Model file for the job. Use its own axes, mm. A direction names the side the tool comes from. Give positions to 0.01 mm unless a question says otherwise; leave off trailing zeros. Loops run counter-clockwise (first coordinate to the right, second up) from the corner with the lowest first, then second, coordinate; pieces in that order, holes last. Notation, with made-up numbers: M -20,-24.5 L 33,-24.5 A16 ccw 33,-8.5 Z; hole C -10,65 d8. An arc over 180 degrees is marked long. Use CSV: the item, a comma, the result in double quotes. Start each with the question number.
(1) Flat gauge pins, fed straight in: P1, Ø20, axis at y = 54, z = 58.5, coming from the -X side; P2, Ø5, axis at y = 65, z = 67, coming from the +X side; P3, Ø6, axis at x = 40.5, y = 64.5, coming from the +Z side. Where does each tip first touch, or does it go through?
(2) Two-plate mould, pull along Y, no slides. Class faces 6 (the face through (50, 0, 50)), 7 (the face through (50, 40, 57)), 8 (the face through (88, 32, 49)), 9 (the face through (80, 5, 50)): pulls with the +Y half, pulls with the -Y half, needs draft (parallel to the pull), parting line crosses it, or undercut.
(3) Slice it at D-D on z = 17.5. List the corners of the cut face in (x, y), and give its area (3 significant figures).
(4) Slice it at B-B on y = 43.5. List the corners of the cut face in (x, z), and give its area (3 significant figures).
(5) Tool access for faces 1 (the face through (50, 60, 57)), 2 (the face through (20, 65, 41)), 3 (the face through (83, 10, 51)), 4 (the face through (80, 64, 41)), 5 (the face through (20, 5, 50)): list every direction of +Z, -Z, +X, -X, +Y, -Y with a clear straight run to the whole face (end or side of a thin tool).
(6) Wall check: line 1 along Y through (x, z) = (34.5, 39); line 2 along X through (y, z) = (60.5, 67.5); line 3 along Z through (x, y) = (50.5, 43.5). Give the ranges that are in metal, low to high. Write a range as from..to.
(7) Slice it at C-C on x = 41. List the corners of the cut face in (y, z).
(8) Slice it at A-A on z = 94. List the corners of the cut face in (x, y), and give its area (3 significant figures).
```python
from build123d import *

# Parameters (mm, degrees)
SKETCH1_W           = 100
SKETCH1_H           = 80
BOSS_EXTRUDE2_DEPTH = 100
SKETCH2_W           = 20
SKETCH2_H           = 10
CUT_EXTRUDE1_DEPTH  = 100
CUT_EXTRUDE2_DEPTH  = 100
SKETCH4_W           = 15
SKETCH4_H           = 10
CUT_EXTRUDE5_DEPTH  = 100
SKETCH7_R           = 35
CUT_EXTRUDE16_DEPTH = 20
BOSS_EXTRUDE3_DEPTH = 40
CUT_EXTRUDE17_DEPTH = 10
SKETCH18_W          = 60
SKETCH18_H          = 20
CUT_EXTRUDE22_DEPTH = 75


with BuildPart() as part:
    # Sketch1 → Boss-Extrude2 (new body)
    with BuildSketch(Plane.XY):
        with Locations((50, 40)):
            Rectangle(SKETCH1_W, SKETCH1_H)
    extrude(amount=BOSS_EXTRUDE2_DEPTH)

    # Sketch2 → Cut-Extrude1 (cut)
    with BuildSketch(Plane.XY):
        Polygon((0, 80), (20, 80), (20, 40), (0, 20), align=None)
        with Locations((10, 5)):
            Rectangle(SKETCH2_W, SKETCH2_H)
        with Locations((90, 5)):
            Rectangle(SKETCH2_W, SKETCH2_H)
        Polygon((80, 80), (100, 80), (100, 20), (80, 40), align=None)
    extrude(amount=CUT_EXTRUDE1_DEPTH, mode=Mode.SUBTRACT)

    # Sketch3 → Cut-Extrude2 (cut)
    with BuildSketch(Plane(origin=(0, 80, 0), x_dir=(1, 0, 0), z_dir=(0, 1, 0))):
        with BuildLine():
            Line((0, 0), (0, -50))
            ThreePointArc((0, -50), (14.644660941, -14.644660941), (50, 0))
            Line((50, 0), (0, 0))
        make_face()
        with BuildLine():
            Line((100, 0), (50, 0))
            ThreePointArc((50, 0), (85.355339059, -14.644660941), (100, -50))
            Line((100, -50), (100, 0))
        make_face()
        with BuildLine():
            ThreePointArc((100, -50), (85.355339059, -85.355339059), (50, -100))
            Line((50, -100), (100, -100))
            Line((100, -100), (100, -50))
        make_face()
        with BuildLine():
            ThreePointArc((50, -100), (14.644660941, -85.355339059), (0, -50))
            Line((0, -50), (0, -100))
            Line((0, -100), (50, -100))
        make_face()
    extrude(amount=-CUT_EXTRUDE2_DEPTH, mode=Mode.SUBTRACT)

    # Sketch4 → Cut-Extrude5 (cut)
    with BuildSketch(Plane(origin=(0, 0, 0), x_dir=(0, 0, -1), z_dir=(1, 0, 0))):
        with Locations((-7.5, 5)):
            Rectangle(SKETCH4_W, SKETCH4_H)
        with Locations((-92.5, 5)):
            Rectangle(SKETCH4_W, SKETCH4_H)
    extrude(amount=CUT_EXTRUDE5_DEPTH, mode=Mode.SUBTRACT)

    # Sketch7 → Cut-Extrude16 (cut)
    with BuildSketch(Plane(origin=(0, 60, 0), x_dir=(1, 0, 0), z_dir=(0, 1, 0))):
        with BuildLine():
            Line((15, -85), (50, -85))
            ThreePointArc((50, -85), (25.251262658, -74.748737342), (15, -50))
            Line((15, -50), (15, -85))
        make_face()
        with BuildLine():
            ThreePointArc((50, -15), (74.748737342, -25.251262658), (85, -50))
            Line((85, -50), (85, -15))
            Line((85, -15), (50, -15))
        make_face()
        with BuildLine():
            ThreePointArc((85, -50), (74.748737342, -74.748737342), (50, -85))
            Line((50, -85), (85, -85))
            Line((85, -85), (85, -50))
        make_face()
        with BuildLine():
            Line((15, -15), (15, -50))
            ThreePointArc((15, -50), (25.251262658, -25.251262658), (50, -15))
            Line((50, -15), (15, -15))
        make_face()
        with Locations((50, -50)):
            Circle(SKETCH7_R)
    extrude(amount=-CUT_EXTRUDE16_DEPTH, mode=Mode.SUBTRACT)

    # Sketch8 → Boss-Extrude3 (add)
    with BuildSketch(Plane(origin=(0, 80, 0), x_dir=(1, 0, 0), z_dir=(0, 1, 0))):
        with BuildLine():
            ThreePointArc((20, -31.972243623), (32.765898242, -19.537141687), (50, -15))
            Line((50, -15), (20, -15))
            Line((20, -15), (20, -31.972243623))
        make_face()
        with BuildLine():
            Line((80, -15), (50, -15))
            ThreePointArc((50, -15), (67.234101758, -19.537141687), (80, -31.972243623))
            Line((80, -31.972243623), (80, -15))
        make_face()
        with BuildLine():
            ThreePointArc((50, -85), (32.765898242, -80.462858313), (20, -68.027756377))
            Line((20, -68.027756377), (20, -85))
            Line((20, -85), (50, -85))
        make_face()
        with BuildLine():
            Line((80, -85), (80, -68.027756377))
            ThreePointArc((80, -68.027756377), (67.234101758, -80.462858313), (50, -85))
            Line((50, -85), (80, -85))
        make_face()
    extrude(amount=-BOSS_EXTRUDE3_DEPTH)

    # Sketch9 → Cut-Extrude17 (cut)
    with BuildSketch(Plane.XZ):
        with BuildLine():
            Line((20, 85), (20, 68.027756377))
            ThreePointArc((20, 68.027756377), (32.765898242, 80.462858313), (50, 85))
            Line((50, 85), (20, 85))
        make_face()
        with BuildLine():
            Line((80, 85), (50, 85))
            ThreePointArc((50, 85), (67.234101758, 80.462858313), (80, 68.027756377))
            Line((80, 68.027756377), (80, 85))
        make_face()
        with BuildLine():
            ThreePointArc((80, 31.972243623), (67.234101758, 19.537141687), (50, 15))
            Line((50, 15), (80, 15))
            Line((80, 15), (80, 31.972243623))
        make_face()
        with BuildLine():
            ThreePointArc((50, 15), (32.765898242, 19.537141687), (20, 31.972243623))
            Line((20, 31.972243623), (20, 15))
            Line((20, 15), (50, 15))
        make_face()
    extrude(amount=-CUT_EXTRUDE17_DEPTH, mode=Mode.SUBTRACT)

    # Sketch18 → Cut-Extrude22 (cut)
    with BuildSketch(Plane.XY.offset(50)):
        with Locations((50, 50)):
            Rectangle(SKETCH18_W, SKETCH18_H)
    extrude(amount=CUT_EXTRUDE22_DEPTH, mode=Mode.SUBTRACT)


solid = part.part
```
Reply:
1,P1,"stops at x = 20"
1,P2,"stops at x = 80"
1,P3,"stops at z = 99.58"
2,face 6,"pulls with the -Y half"
2,face 7,"undercut"
2,face 8,"pulls with the +Y half"
2,face 9,"needs draft"
3,outline,"M 12,10 L 37.01,10 L 37.01,0 L 62.99,0 L 62.99,10 L 88,10 L 88,32 L 80,40 L 80,80 L 20,80 L 20,40 L 12,32 Z; hole M 37.01,40 L 62.99,40 L 62.99,60 L 37.01,60 Z"
3,area,"4,360 mm^2"
4,outline,"M 20,10 A50 ccw 80,10 L 80,31.97 A35 cw 20,31.97 Z"
4,area,"1,010 mm^2"
5,face 1,"+Z"
5,face 2,"+Z, -Z, -X, +Y"
5,face 3,"-Y"
5,face 4,"+Z, -Z, +X, +Y"
5,face 5,"+Z, -Z, -X, -Y"
6,line 1,"y = 0..40, 60..80"
6,line 2,"x = 20..80"
6,line 3,"z = 0..15"
7,outline,"M 0,16.18 L 10,16.18 L 10,0.82 L 80,0.82 L 80,99.18 L 60,99.18 L 60,16.18 L 40,16.18 L 40,99.18 L 10,99.18 L 10,83.82 L 0,83.82 Z"
8,outline,"M 26.25,10 L 73.75,10 L 73.75,40 L 26.25,40 Z; M 26.25,60 L 73.75,60 L 73.75,80 L 26.25,80 Z"
8,area,"2,370 mm^2"
